```python
from build123d import *

# Parameters (mm, degrees)
SKETCH1_R           = 1.3375
BOSS_EXTRUDE1_DEPTH = 2.275


with BuildPart() as part:
    # Sketch1 → Boss-Extrude1 (new body)
    with BuildSketch(Plane.XY):
        Polygon((0, 3.175426481), (-2.75, 1.58771324), (-2.75, -1.58771324), (0, -3.175426481), (2.75, -1.58771324), (2.75, 1.58771324), align=None)
        Circle(SKETCH1_R, mode=Mode.SUBTRACT)
    extrude(amount=BOSS_EXTRUDE1_DEPTH)

    # Sketch2 → Cut-Revolve1 (revolve, cut)
    with BuildSketch(Plane(origin=(0, 0, 0), x_dir=(0, 0, -1), z_dir=(1, 0, 0))):
        Polygon((-2.275, 1.3375), (-2.275, 1.5), (-2.1125, 1.3375), align=None)
        Polygon((-2.275, 3.175426481), (-2.275, 2.75), (-2.029379907, 3.175426481), align=None)
        Polygon((-0.245620093, 3.175426481), (0, 3.175426481), (0, 2.75), align=None)
        Polygon((-0.1625, 1.3375), (0, 1.3375), (0, 1.5), align=None)
    revolve(axis=Axis((0, 0, 0), (0, 0, 1)), mode=Mode.SUBTRACT)


solid = part.part
```
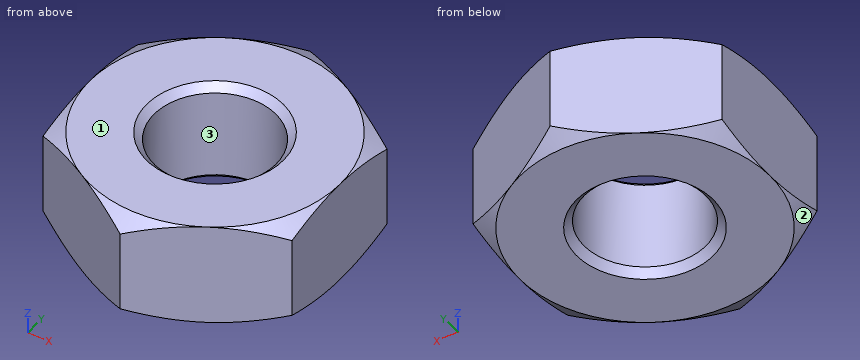
Work out the finished part from the listing and answer in its coordinate system (mm). Face numbers are marked on the shaded views. Give positions to 0.01 mm unless a question says otherwise; leave off trailing zeros. One line per question, with ' | ' between items. Start each with the question number.
1) This flat-tipped pin is pushed along its axis until it touches: pin 1 (2 mm diameter, centred on x = 0, y = 0, fed in from +Z). Where does it stop, or does it pass through?
2) Determine the mould class of the marked faces 1, 2 and 3 for opening direction X: +X half, -X half, draft (parallel to the pull), parting line (faces both ways), or undercut.
3) Straight lines are drawn through the part: L1, parallel to X at y = -1, z = 1.3; L2, parallel to Y at x = -0.3, z = 0.3; L3, parallel to Y at x = -0.9, z = 0.8. For each, find the intervals that lie inside material, in ascending order.
Resolved:
1) pin 1: through
2) face 1: draft | face 2: -X half | face 3: undercut
3) L1: -2.75 to -0.89, 0.89 to 2.75 | L2: -3 to -1.3, 1.3 to 3 | L3: -2.66 to -0.99, 0.99 to 2.66
